Geometry: final body of the model. Coordinates: model frame, mm. Face numbers are marked on the shaded views. A direction names the side the tool comes from. Give positions to 0.01 mm unless a question says otherwise; leave off trailing zeros. Loops run counter-clockwise (first coordinate to the right, second up) from the corner with the lowest first, then second, coordinate; pieces in that order, holes last. Notation, with made-up numbers: (19.25, 58) -> (23.25, 58) arc R21 ccw to (23.25, 81) -> close; hole circle Ø5 at (57.5, -24.75). An arc over 180 degrees is marked (long way). One line per question, with ' | ' between items. Start each with the question number.
Item 1: Section A-A on x = 0. Return loops of the section in (y, z), then the cut area to 4 significant figures.
Item 2: Section C-C on z = 1.9. Give the number of separate pieces and of enclosed holes in the cut face, then the cut area to 3 significant figures.
Item 3: Material intervals for line 1 along X through (y, z) = (-20, 2.25); line 2 along Y through (x, z) = (1.5, 1.8); line 3 along Y through (x, z) = (-24.5, 0.7), sorted ascending. Write a range as [from, to].
Item 4: Mould query, pull axis Y, two halves, no side actions, for the marked faces 1, 2 and 3. Classes: released by +Y, released by -Y, zero draft, split by the parting line, or undercut.
Item 5: Pin query (flat end, axial travel): P1, Ø1.5, axis at x = 8, z = 4, coming from the -Y side; P2, Ø6, axis at x = 10.52, y = 25.41, coming from the +Z side; P3, Ø1, axis at y = 1.5, z = 0.5, coming from the +X side. Return the tip coordinate at first contact, or that it passes through.
Item 6: Set-up query: the marked faces 4, 5 and 6. Return all of +Z, -Z, +X, -X, +Y, -Y with unobstructed straight access to the full face (end or side cutting, diameter ignored); none if empty.
Item 7: Section B-B on y = 16. Return loops of the section in (x, z).
from build123d import *

# Parameters (mm, degrees)
SKETCH_1_R                     = 30.999999999999996
EXTRUDE_1_DEPTH                = 5
SKETCH_2_R                     = 6
CUT_EXTRUDE_1_DEPTH            = 45.12482294582041
HOLE_WIZARD_M3_1_D             = 3.4
HOLE_WIZARD_M3_1_2_D           = 3.6
HOLE_WIZARD_M3_1_2_CSINK_D     = 7.3
HOLE_WIZARD_M3_1_2_CSINK_ANGLE = 90
PATTERN_CIRCULAR_1_COUNT       = 8
HOLE_WIZARD_M3_2_D             = 3.4
PATTERN_CIRCULAR_2_COUNT       = 3
CUT_EXTRUDE_4_DEPTH            = 45.124823097662386
FILLET_1_R                     = 2
PATTERN_CIRCULAR_5_DEPTH       = 5
SKETCH_13_R                    = 1.9
SKETCH_13_R_2                  = 1.8999999999999984
CUT_EXTRUDE_5_DEPTH            = 45.124823097662386
CUT_EXTRUDE_6_DEPTH            = 1.5
FILLET_2_R                     = 1


# Read off the part's stored shape, not the designer's step: 円形ﾊﾟﾀｰﾝ5
with BuildPart() as part:
    # ｽｹｯﾁ1 → ﾎﾞｽ - 押し出し1 (new body)
    with BuildSketch(Plane.XY):
        Circle(SKETCH_1_R)
    extrude(amount=EXTRUDE_1_DEPTH)

    # ｽｹｯﾁ2 → ｶｯﾄ - 押し出し1 (cut, through all)
    with BuildSketch(Plane.XY.offset(5)):
        Circle(SKETCH_2_R)
    extrude(amount=-CUT_EXTRUDE_1_DEPTH, mode=Mode.SUBTRACT)

    # Hole Wizard M3 _1 (through all)
    with Locations(Plane.XY.offset(5)):
        with Locations((0, 27.5)):
            hole_wizard_m3_1 = Hole(HOLE_WIZARD_M3_1_D / 2)

    # Hole Wizard M3 _1 2 (through all)
    with Locations(Plane.XY.offset(5)):
        with Locations((10.52379439, 25.406687144)):
            hole_wizard_m3_1_2 = CounterSinkHole(HOLE_WIZARD_M3_1_2_D / 2, HOLE_WIZARD_M3_1_2_CSINK_D / 2, counter_sink_angle=HOLE_WIZARD_M3_1_2_CSINK_ANGLE)

    # 円形ﾊﾟﾀｰﾝ1: Hole Wizard M3 _1, Hole Wizard M3 _1 2 ×8 about axis
    pattern_circular_1_axis = Axis((-2.28e-14, 6.09e-15, 0), (0, 0, 1))
    add([hole_wizard_m3_1.rotate(pattern_circular_1_axis, i * 360 / PATTERN_CIRCULAR_1_COUNT) for i in range(1, PATTERN_CIRCULAR_1_COUNT)], mode=Mode.SUBTRACT)
    add([hole_wizard_m3_1_2.rotate(pattern_circular_1_axis, i * 360 / PATTERN_CIRCULAR_1_COUNT) for i in range(1, PATTERN_CIRCULAR_1_COUNT)], mode=Mode.SUBTRACT)

    # M3 すきま穴2 (through all)
    with Locations(Plane.XY.offset(5)):
        with Locations((0, 16)):
            hole_wizard_m3_2 = Hole(HOLE_WIZARD_M3_2_D / 2)

    # 円形ﾊﾟﾀｰﾝ2: M3 すきま穴2 ×3 about axis
    pattern_circular_2_axis = Axis((6.2e-16, -9.3e-16, 0), (0, 0, 1))
    for i in range(1, PATTERN_CIRCULAR_2_COUNT):
        add(hole_wizard_m3_2.rotate(pattern_circular_2_axis, i * 360 / PATTERN_CIRCULAR_2_COUNT), mode=Mode.SUBTRACT)

    # ｽｹｯﾁ12 → ｶｯﾄ - 押し出し4 (cut, through all)
    with BuildSketch(Plane.XY.offset(5)):
        with BuildLine():
            Line((-8.356238925925028, -9.958577760546698), (-15.42690263247697, -18.38506663485545))
            ThreePointArc((-15.42690263247697, -18.38506663485545), (1.036e-14, -23.999999999999986), (15.426902632476974, -18.38506663485544))
            Line((15.426902632476974, -18.38506663485544), (8.356238925925028, -9.958577760546694))
            ThreePointArc((8.356238925925028, -9.958577760546694), (8e-16, -12.999999999999998), (-8.356238925925028, -9.958577760546698))
        make_face()
    extrude(amount=-CUT_EXTRUDE_4_DEPTH, mode=Mode.SUBTRACT)

    # ﾌｨﾚｯﾄ1
    fillet_1_edges = [part.edges().sort_by_distance(p)[0] for p in [
        (15.426902632476974, -18.38506663485544, 2.5),
        (-15.42690263247697, -18.38506663485545, 2.5),
        (-8.35623892592503, -9.9585777605467, 2.5),
        (8.35623892592503, -9.958577760546696, 2.5),
    ]]
    fillet(fillet_1_edges, radius=FILLET_1_R)

    # 円形ﾊﾟﾀｰﾝ5 outline → 円形ﾊﾟﾀｰﾝ5 (cut)
    with BuildSketch(Plane.XY):
        with BuildLine():
            ThreePointArc((21.576056845, -3.804440959), (23.143863501, -3.419235313), (23.91638531, -2.001627767))
            ThreePointArc((23.91638531, -2.001627767), (20.784609691, 12), (10.22473216, 21.713011128))
            ThreePointArc((10.22473216, 21.713011128), (8.610787108, 21.752791391), (7.493285905, 20.587633821))
            Line((7.493285905, 20.587633821), (5.084494964, 13.969535102))
            ThreePointArc((5.084494964, 13.969535102), (5.098839949, 12.563258813), (6.035362845, 11.514095507))
            ThreePointArc((6.035362845, 11.514095507), (11.258330249, 6.5), (12.989180633, -0.530270209))
            ThreePointArc((12.989180633, -0.530270209), (13.429521261, -1.865904481), (14.640219759, -2.581465747))
            Line((14.640219759, -2.581465747), (21.576056845, -3.804440959))
        make_face()
        with BuildLine():
            ThreePointArc((-7.493285905, 20.587633821), (-8.610787108, 21.752791391), (-10.22473216, 21.713011128))
            ThreePointArc((-10.22473216, 21.713011128), (-20.784609691, 12), (-23.91638531, -2.001627767))
            ThreePointArc((-23.91638531, -2.001627767), (-23.143863501, -3.419235313), (-21.576056845, -3.804440959))
            Line((-21.576056845, -3.804440959), (-14.640219759, -2.581465747))
            ThreePointArc((-14.640219759, -2.581465747), (-13.429521261, -1.865904481), (-12.989180633, -0.530270209))
            ThreePointArc((-12.989180633, -0.530270209), (-11.258330249, 6.5), (-6.035362845, 11.514095507))
            ThreePointArc((-6.035362845, 11.514095507), (-5.098839949, 12.563258813), (-5.084494964, 13.969535102))
            Line((-5.084494964, 13.969535102), (-7.493285905, 20.587633821))
        make_face()
    extrude(amount=PATTERN_CIRCULAR_5_DEPTH, mode=Mode.SUBTRACT)

    # ｽｹｯﾁ13 → ｶｯﾄ - 押し出し5 (cut, through all)
    with BuildSketch(Plane.XY.offset(5)):
        with Locations((-8.999999999999998, 5.499999999999997)):
            Circle(SKETCH_13_R)
        with Locations((9.000000000000002, 5.499999999999997)):
            Circle(SKETCH_13_R_2)
        with Locations((-8.999999999999998, -5.500000000000003)):
            Circle(SKETCH_13_R)
        with Locations((9.000000000000002, -5.500000000000003)):
            Circle(SKETCH_13_R_2)
    extrude(amount=-CUT_EXTRUDE_5_DEPTH, mode=Mode.SUBTRACT)

    # ｽｹｯﾁ14 → ｶｯﾄ - 押し出し6 (cut)
    with BuildSketch(Plane.XY.offset(5)):
        with BuildLine():
            Line((-9.555724795524648, -11.388069354908032), (-3.8567256581192475, -4.596266658713859))
            ThreePointArc((-3.8567256581192475, -4.596266658713859), (3.7e-16, -6.000000000000001), (3.8567256581192484, -4.59626665871386))
            Line((3.8567256581192484, -4.59626665871386), (9.55572479552465, -11.38806935490803))
            ThreePointArc((9.55572479552465, -11.38806935490803), (9.1e-16, -14.866068747318506), (-9.555724795524648, -11.388069354908032))
        make_face()
    extrude(amount=-CUT_EXTRUDE_6_DEPTH, mode=Mode.SUBTRACT)

    # ﾌｨﾚｯﾄ2
    fillet_2_edges = [part.edges().sort_by_distance(p)[0] for p in [
        (-6.706225226821948, -7.992168006810946, 3.5),
        (6.7062252268219495, -7.992168006810945, 3.5),
    ]]
    fillet(fillet_2_edges, radius=FILLET_2_R)


solid = part.part
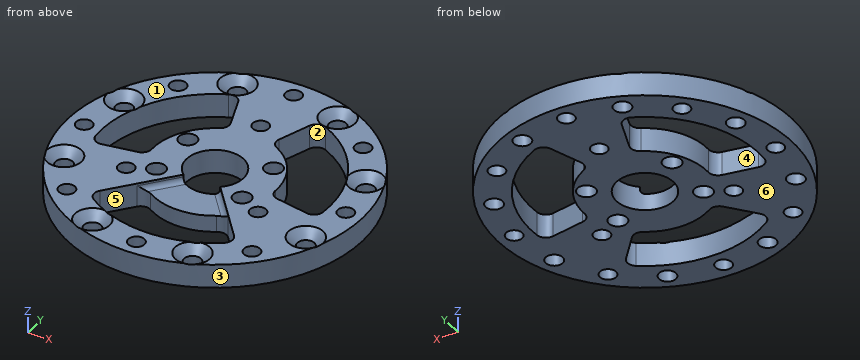
Result sheet:
1) outline: (-31, 0) -> (-29.2, 0) -> (-29.2, 5) -> (-31, 5) -> close; (-25.8, 0) -> (-24, 0) -> (-24, 5) -> (-25.8, 5) -> close; (-13, 0) -> (-6, 0) -> (-6, 3.5) -> (-13, 3.5) -> close; (6, 0) -> (14.3, 0) -> (14.3, 5) -> (6, 5) -> close; (17.7, 0) -> (25.8, 0) -> (25.8, 5) -> (17.7, 5) -> close; (29.2, 0) -> (31, 0) -> (31, 5) -> (29.2, 5) -> close | area: 133.5 mm²
2) separate pieces: 1 | enclosed holes: 27 | area: 1,840 mm²
3) line 1: x = [-23.69, -21.05], [-17.84, -13.27], [13.27, 17.84], [21.05, 23.69] | line 2: y = [-30.96, -28.3], [-26.7, -23.95], [-12.91, -5.81], [5.81, 15.2], [16.8, 26.7], [28.3, 30.96] | line 3: y = [-18.99, -12.08], [-8.97, 8.97], [12.08, 18.99]
4) face 1: zero draft | face 2: undercut | face 3: split by the parting line
5) P1: stops at y = -30.14 | P2: stops at z = 4.36 | P3: stops at x = 30.98
6) face 4: +Z, -Z | face 5: +Z | face 6: -Z, +X, -X, +Y, -Y
7) outline: (-26.55, 0) -> (-17.89, 0) -> (-17.89, 5) -> (-26.55, 5) -> close; (-5.82, 0) -> (-1.7, 0) -> (-1.7, 5) -> (-5.82, 5) -> close; (1.7, 0) -> (5.82, 0) -> (5.82, 5) -> (1.7, 5) -> close; (17.89, 0) -> (26.55, 0) -> (26.55, 5) -> (17.89, 5) -> close
